Autodesk Inventor part; units mm, degrees
ref_plane "YZ Plane" through (0, 0, 0) normal (1, 0, 0) x (0, 1, 0)
ref_plane "XZ Plane" through (0, 0, 0) normal (0, 1, 0) x (-1, 0, 0)
ref_plane "XY Plane" through (0, 0, 0) normal (0, 0, 1) x (1, 0, 0)
sketch "Szkic1" plane through (0, 0, 0) normal (0, 0, 1) x (1, 0, 0)
  line L0 (-30, -30) -> (30, -30)
  line L1 (30, -30) -> (30, 30)
  line L2 (30, 30) -> (-30, 30)
  line L3 (-30, 30) -> (-30, -30)
  line L4 (-30, -30) -> (30, 30) construction
  line L5 (30, -30) -> (-30, 30) construction
  point P0 (0, 0)
  dimension "d0" = 60
  dimension "d1" = 60
extrude "Wyciągnięcie proste1" add sketch "Szkic1" along normal blind 100
sketch "Szkic2" plane through (0, 0, 100) normal (0, 0, 1) x (1, 0, 0)
  circle A0 centre (0, 0) radius 19.05
  dimension "d4" = 38.1
extrude "Wyciągnięcie proste2" add sketch "Szkic2" along normal blind 1.6
sketch "Szkic3" plane through (0, 0, 100) normal (0, 0, 1) x (1, 0, 0)
  line L0 (0, 0) -> (0, 23.57)
  line L1 (30, -30) -> (30, 30)
  line L2 (-30, 30) -> (-30, -30)
  line L3 (0, 0) -> (0, -23.57)
  line L4 (0, -23.57) -> (23.57, -23.57)
  line L5 (0, -23.57) -> (-23.57, -23.57)
  line L6 (0, 23.57) -> (-23.57, 23.57)
  line L7 (0, 23.57) -> (23.57, 23.57)
  circle A0 centre (23.57, 23.57) radius 2.5
  circle A1 centre (-23.57, 23.57) radius 2.5
  circle A2 centre (-23.57, -23.57) radius 2.5
  circle A3 centre (23.57, -23.57) radius 2.5
  dimension "d13" = 47.14
  dimension "d14" = 47.14
  dimension "d15" = 47.14
  dimension "d16" = 5
  dimension "d17" = 5
  dimension "d18" = 5
  dimension "d19" = 5
extrude "Wyciągnięcie proste3" cut sketch "Szkic3" against normal up to next
sketch "Szkic4" plane through (0, 0, 0) normal (0, 0, -1) x (-1, 0, 0)
  circle A0 centre (23.57, -23.57) radius 2.5
  circle A1 centre (-23.57, 23.57) radius 2.5
  circle A2 centre (23.57, 23.57) radius 2.5
  circle A3 centre (-23.57, -23.57) radius 2.5
  line L0 (30, -30) -> (-30, -30)
  line L1 (30, 30) -> (30, -30)
  line L2 (-30, 30) -> (30, 30)
  line L3 (-30, -30) -> (-30, 30)
  line L4 (-30, -30) -> (-30, 30)
  line L5 (-17, -17) -> (-17, -30)
  line L6 (17, -17) -> (17, -30)
  line L7 (30, 30) -> (30, -30)
  line L8 (-17, -17) -> (-30, -17)
  line L9 (17, 17) -> (30, 17)
  line L10 (-17, 17) -> (-17, 30)
  line L11 (-17, 17) -> (-30, 17)
  line L12 (17, 17) -> (17, 30)
  line L13 (17, -17) -> (30, -17)
  point P0 (0, 0)
extrude "Wyciągnięcie proste4" cut sketch "Szkic4" against normal blind 96 contours L0 L6 L13 L1 | L0 L3 L8 L5 | L9 L12 L2 L1 | L3 L2 L10 L11
sketch "Szkic5" plane through (0, 0, 101.6) normal (0, 0, 1) x (1, 0, 0)
  circle A0 centre (0, 0) radius 3.75
  dimension "d25" = 7.5
extrude "Wyciągnięcie proste5" add sketch "Szkic5" along normal blind 22.5
sketch "Szkic6" plane through (-30, 30, 100) normal (0, 1, 0) x (1, 0, 0)
  line L0 (13, 100) -> (13, 4)
  line L1 (13, 4) -> (0, 4)
  line L2 (0, 4) -> (0, 0)
  line L3 (60, 0) -> (0, 0)
  line L4 (60, 4) -> (60, 0)
  line L5 (60, 4) -> (47, 4)
  line L6 (47, 4) -> (47, 100)
  line L7 (47, 100) -> (13, 100)
  line L8 (13, 4) -> (47, 4)
  line L9 (13, 100) -> (13, 4)
  line L10 (13, 100) -> (13, 96)
  line L11 (13, 96) -> (47, 96)
  point P0 (30, 100)
  dimension "d28" = 4
extrude "Wyciągnięcie proste6" cut sketch "Szkic6" against normal blind 1 contours L11 L6 L8 L0
sketch "Szkic7" plane through (-30, -30, 100) normal (-1, 0, 0) x (0, 0, 1)
  line L0 (-4, 47) -> (-100, 47)
  line L1 (-100, 47) -> (-100, 13)
  line L2 (-100, 13) -> (-4, 13)
  line L3 (-4, 13) -> (-4, 0)
  line L4 (-4, 0) -> (0, 0)
  line L5 (0, 60) -> (0, 0)
  line L6 (-4, 60) -> (0, 60)
  line L7 (-4, 60) -> (-4, 47)
  line L8 (-100, 47) -> (-4, 47)
  line L9 (-100, 13) -> (-4, 13)
  line L10 (-4, 47) -> (-4, 13)
  line L11 (-100, 47) -> (-100, 13)
  line L12 (-96, 13) -> (-96, 47)
  point P0 (-100, 30)
sketch "Szkic8" plane through (-30, -30, 100) normal (0, -1, 0) x (1, 0, 0)
  line L0 (13, -4) -> (13, -100)
  line L1 (13, -100) -> (47, -100)
  line L2 (47, -100) -> (47, -4)
  line L3 (47, -4) -> (60, -4)
  line L4 (60, -4) -> (60, 0)
  line L5 (0, 0) -> (60, 0)
  line L6 (0, -4) -> (0, 0)
  line L7 (0, -4) -> (13, -4)
  line L8 (47, -4) -> (13, -4)
  line L9 (13, -4) -> (47, -4)
  line L10 (47, -100) -> (47, -96)
  line L11 (47, -100) -> (47, -4)
  line L12 (47, -96) -> (13, -96)
  point P0 (30, -100)
  dimension "d34" = 4
sketch "Szkic9" plane through (30, -30, 100) normal (1, 0, 0) x (0, 0, -1)
  line L0 (4, 13) -> (100, 13)
  line L1 (100, 13) -> (100, 47)
  line L2 (100, 47) -> (4, 47)
  line L3 (4, 47) -> (4, 60)
  line L4 (4, 60) -> (0, 60)
  line L5 (0, 0) -> (0, 60)
  line L6 (4, 0) -> (0, 0)
  line L7 (4, 0) -> (4, 13)
  line L8 (4, 47) -> (4, 13)
  line L9 (4, 13) -> (4, 47)
  line L10 (100, 47) -> (100, 60)
  line L11 (100, 47) -> (96, 47)
  line L12 (100, 47) -> (4, 47)
  line L13 (96, 47) -> (96, 13)
  line L14 (100, 13) -> (4, 13)
  point P0 (100, 30)
  dimension "d37" = 4
extrude "Wyciągnięcie proste10" cut sketch "Szkic8" against normal blind 1 contours L8 L2 L12 L0
extrude "Wyciągnięcie proste11" cut sketch "Szkic7" against normal blind 1 contours L10 L2 L12 L0
extrude "Wyciągnięcie proste12" cut sketch "Szkic9" against normal blind 1 contours L8 L2 L13 L0
sketch "Szkic10" plane through (-30, 17, 0) normal (0, 1, 0) x (1, 0, 0)
  line L0 (1, -4) -> (1, -96)
  line L1 (1, -96) -> (13, -96)
  line L2 (13, -4) -> (13, -96)
  line L3 (1, -4) -> (1, -96)
  line L4 (1, -4) -> (13, -4)
  point P0 (30, 0)
extrude "Wyciągnięcie proste13" cut sketch "Szkic10" against normal blind 1
sketch "Szkic11" plane through (-17, 17, 0) normal (-1, 0, 0) x (0, 0, 1)
  line L0 (4, 0) -> (4, -1)
  line L1 (4, -1) -> (96, -1)
  line L2 (96, -1) -> (96, 12)
  line L3 (96, 12) -> (4, 12)
  line L4 (96, 12) -> (4, 12)
  line L5 (4, 12) -> (4, 0)
  point P0 (0, -17)
extrude "Wyciągnięcie proste14" cut sketch "Szkic11" against normal blind 1
sketch "Szkic12" plane through (17, 17, 0) normal (0, 1, 0) x (1, 0, 0)
  line L0 (12, -96) -> (12, -4)
  line L1 (0, -4) -> (0, -96)
  line L2 (0, -96) -> (12, -96)
  line L3 (12, -4) -> (0, -4)
  point P0 (-17, 0)
extrude "Wyciągnięcie proste15" cut sketch "Szkic12" against normal blind 1
sketch "Szkic13" plane through (17, 17, 0) normal (1, 0, 0) x (0, 0, -1)
  line L0 (-4, 12) -> (-96, 12)
  line L1 (-96, 12) -> (-96, -1)
  line L2 (-96, -1) -> (-4, -1)
  line L3 (-4, 0) -> (-4, -1)
  line L4 (-4, -1) -> (-4, 12)
  line L5 (-4, 0) -> (-4, 12)
  point P0 (0, -17)
extrude "Wyciągnięcie proste16" cut sketch "Szkic13" against normal blind 1
sketch "Szkic14" plane through (17, -17, 0) normal (0, -1, 0) x (1, 0, 0)
  line L0 (12, 4) -> (12, 96)
  line L1 (12, 96) -> (0, 96)
  line L2 (0, 4) -> (0, 96)
  line L3 (0, 4) -> (12, 4)
  line L4 (-1, 4) -> (-1, 96)
  point P0 (-17, 0)
extrude "Wyciągnięcie proste17" cut sketch "Szkic14" against normal blind 1
sketch "Szkic15" plane through (17, -30, 0) normal (1, 0, 0) x (0, 0, -1)
  line L0 (-96, 1) -> (-4, 1)
  line L1 (-4, 13) -> (-4, 14)
  line L2 (-4, 14) -> (-96, 14)
  line L3 (-96, 14) -> (-96, 1)
  line L4 (-4, 1) -> (-96, 1)
  line L5 (-4, 1) -> (-4, 13)
  point P0 (0, 30)
extrude "Wyciągnięcie proste18" cut sketch "Szkic15" against normal blind 1
sketch "Szkic16" plane through (-30, -17, 0) normal (0, -1, 0) x (1, 0, 0)
  line L0 (1, 96) -> (1, 4)
  line L1 (13, 4) -> (13, 96)
  line L2 (13, 96) -> (1, 96)
  line L3 (1, 4) -> (14, 4)
  line L4 (13, 4) -> (1, 4)
  point P0 (30, 0)
extrude "Wyciągnięcie proste19" cut sketch "Szkic16" against normal blind 1
sketch "Szkic17" plane through (-17, -30, 0) normal (-1, 0, 0) x (0, 0, 1)
  line L0 (4, 1) -> (96, 1)
  line L1 (96, 1) -> (96, 14)
  line L2 (96, 14) -> (4, 14)
  line L3 (4, 13) -> (4, 14)
  line L4 (4, 14) -> (4, 1)
  line L5 (4, 13) -> (4, 1)
  point P0 (0, 30)
extrude "Wyciągnięcie proste20" cut sketch "Szkic17" against normal blind 1
fillet "Zaokrąglenie1" radius 5 28 edges at (-30, 30, 98) (30, 30, 98) (30, -30, 98) (-30, -30, 98) (-16, -16, 50) (-29, -16, 50) (-16, -29, 50) (16, -29, 50) (16, -16, 50) (29, -16, 50) (29, 16, 50) (16, 16, 50) (16, 29, 50) (-16, 29, 50) (-16, 16, 50) (-29, 16, 50) (-30, 17, 2) (-17, 17, 2) (-17, 30, 2) (17, 30, 2) (17, 17, 2) (30, 17, 2) (30, -17, 2) (17, -17, 2) (17, -30, 2) (-17, -30, 2) (-17, -17, 2) (-30, -17, 2)
properties part number "Silnik krokowy SM 60 100-4004AF - 4Nm"
Here's how the part is built. I have some questions about the finished solid (model axes, mm). A direction names the side the tool comes from. Coordinates: 2 decimals unless noted, no trailing zeros. Write each loop counter-clockwise with the first axis right and the second up, starting at its lowest first coordinate (ties: lowest second). Pieces come first, ordered by that corner, then holes. Notation, with made-up numbers: (27.25, 30.5) - (42.25, 30.5) arc R32 cw to (42.25, 63.5) - close; hole circle Ø2 at (34.5, -4). An arc over 180 degrees is marked (long way). One line per item, written item: value.
1) Suppose I cut it at A-A on x = 0. Write out the boundary of the cut face in (y, z), and give its area (3 significant figures).
Model answer:
outline: (-30, 0) - (30, 0) - (30, 4) - (29, 4) - (29, 96) - (30, 96) - (30, 100) - (19.05, 100) - (19.05, 101.6) - (3.75, 101.6) - (3.75, 124.1) - (-3.75, 124.1) - (-3.75, 101.6) - (-19.05, 101.6) - (-19.05, 100) - (-30, 100) - (-30, 96) - (-29, 96) - (-29, 4) - (-30, 4) - close
area: 6,050 mm²
2) I'm going to push flat-ended pins straight in: P1, Ø1, axis at y = -10.5, z = 83, coming from the -X side; P2, Ø0.9, axis at x = 24, z = 1, coming from the -Y side; P3, Ø0.9, axis at x = 22, z = 42, coming from the -Y side; P4, Ø4, axis at x = -13.5, y = -13, coming from the -Z side. Where does each tip first touch, or does it pass through?
Model answer:
P1: stops at x = -29
P2: stops at y = -17
P3: stops at y = -16
P4: stops at z = 0
3) I need wall thicknesses on line 1 along Y through (x, z) = (-23.57, 98.7); line 2 along Z through (x, y) = (18.5, -17); line 3 along X through (y, z) = (23, 98). Which ranges of each line are inside material? Lowest first, please.
Model answer:
line 1: y = -30 to -26.07, -21.07 to 21.07, 26.07 to 30
line 2: z = 0 to 4, 96 to 100
line 3: x = -30 to -26, -21.14 to 21.14, 26 to 30
4) On a 3-axis mill with a long thin cutter (end or side, diameter ignored), from which of +Z, -Z, +X, -X, +Y, -Y can I reach the whole of each face in a straight line? I mean faces 1 (the cylindrical face through (15, -27, 49)), 2 (the flat face through (18, 20, 96)), 3 (the flat face through (23, 17, 2)), 4 (the cylindrical face through (27, 15, 49)). Say none if no direction works.
Model answer:
face 1: +X, -Y
face 2: none
face 3: -Z, +X, +Y
face 4: +X, +Y
5) Suppose I cut it at C-C on y = -2. Write out the boundary of the cut face in (x, z).
Model answer:
outline: (-30, 0) - (30, 0) - (30, 4) - (29, 4) - (29, 96) - (30, 96) - (30, 100) - (18.94, 100) - (18.94, 101.6) - (3.17, 101.6) - (3.17, 124.1) - (-3.17, 124.1) - (-3.17, 101.6) - (-18.94, 101.6) - (-18.94, 100) - (-30, 100) - (-30, 96) - (-29, 96) - (-29, 4) - (-30, 4) - close
6) Suppose I cut it at B-B on z = 72.5. Write out the boundary of the cut face in (x, y), and give its area (3 significant figures).
Model answer:
outline: (-29, -11) arc R5 ccw to (-24, -16) - (-21, -16) arc R5 cw to (-16, -21) - (-16, -24) arc R5 ccw to (-11, -29) - (11, -29) arc R5 ccw to (16, -24) - (16, -21) arc R5 cw to (21, -16) - (24, -16) arc R5 ccw to (29, -11) - (29, 11) arc R5 ccw to (24, 16) - (21, 16) arc R5 cw to (16, 21) - (16, 24) arc R5 ccw to (11, 29) - (-11, 29) arc R5 ccw to (-16, 24) - (-16, 21) arc R5 cw to (-21, 16) - (-24, 16) arc R5 ccw to (-29, 11) - close
area: 2,670 mm²
7) We'd pull the mould along X, two halves only. Please class faces 5 (the cylindrical face through (-27, -15, 49)), 6 (the cylindrical face through (21.586, -25.091, 98.028)), 7 (the cylindrical face through (18, 17, 49)): pulls with the +X half, pulls with the -X half, needs draft (parallel to the pull), parting line crosses it, or undercut.
Model answer:
face 5: pulls with the -X half
face 6: undercut
face 7: pulls with the +X half
